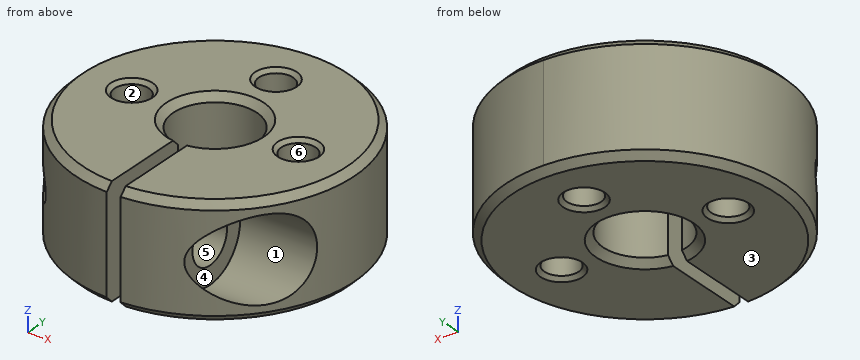
Autodesk Inventor part; units mm, degrees
ref_plane "to_bolt_XY" through (4, -6, 0) normal (1, 0, 0) x (0, 0, -1)
ref_plane "to_bolt_YZ" through (4, -6, 0) normal (0, 0, -1) x (0, 1, 0)
ref_plane "to_bolt_ZX" through (4, -6, 0) normal (0, 1, 0) x (1, 0, 0)
sketch "Sketch_14" plane through (0, 0, 0) normal (1, 0, 0) x (0, 1, 0)
  line L0 (0, -4) -> (0, 4)
  line L1 (0, 4) -> (9.5, 4)
  line L2 (9.5, 4) -> (10, 3.5)
  line L3 (10, 3.5) -> (10, -3.5)
  line L4 (10, -3.5) -> (9.5, -4)
  line L5 (9.5, -4) -> (0, -4)
  line L6 (0, -4) -> (0, 4)
revolve "Revolution1" add sketch "Sketch_14" angle 360 about axis through (0, 0, -4) along (0, 0, -1)
sketch "Sketch_15" plane through (0, 0, 0) normal (1, 0, 0) x (0, 1, 0)
  line L0 (0, -4) -> (0, 4)
  line L1 (0, 4) -> (3.5, 4)
  line L2 (3.5, 4) -> (3, 3.5)
  line L3 (3, 3.5) -> (3, -3.5)
  line L4 (3, -3.5) -> (3.5, -4)
  line L5 (3.5, -4) -> (0, -4)
  line L6 (0, -4) -> (0, 4)
revolve "Revolution2" cut sketch "Sketch_15" angle 360 about axis through (0, 0, -4) along (0, 0, -1)
sketch "Sketch_16" plane through (0, 0, 0) normal (0, 0, 1) x (1, 0, 0)
  arc A0 (-0.5, -10.9886) -> (0.5, -10.9886) centre (0, 0) ccw
  line L0 (0.5, -10.9886) -> (0.5, 0)
  line L1 (0.5, 0) -> (-0.5, 0)
  line L2 (-0.5, 0) -> (-0.5, -10.9886)
extrude "Extrusion1" cut sketch "Sketch_16" along normal mid plane 8
sketch "Sketch_18" plane through (6, 0, 0) normal (1, 0, 0) x (0, 0, -1)
  line L0 (4, 0) -> (-4, 0)
  line L1 (-4, 0) -> (-4, 1.5)
  line L2 (-4, 1.5) -> (-3.7295, 1.2295)
  line L3 (-3.7295, 1.2295) -> (3.7295, 1.2295)
  line L4 (3.7295, 1.2295) -> (4, 1.5)
  line L5 (4, 1.5) -> (4, 0)
  line L6 (4, 0) -> (-4, 0)
revolve "Revolution3" cut sketch "Sketch_18" angle 360 about axis through (6, 0, -4) along (0, 0, -1)
thread "Thread1"
sketch "Sketch_20" plane through (-6, 0, 0) normal (1, 0, 0) x (0, 0, -1)
  line L0 (4, 0) -> (-4, 0)
  line L1 (-4, 0) -> (-4, 1.5)
  line L2 (-4, 1.5) -> (-3.7295, 1.2295)
  line L3 (-3.7295, 1.2295) -> (3.7295, 1.2295)
  line L4 (3.7295, 1.2295) -> (4, 1.5)
  line L5 (4, 1.5) -> (4, 0)
  line L6 (4, 0) -> (-4, 0)
revolve "Revolution4" cut sketch "Sketch_20" angle 360 about axis through (-6, 0, -4) along (0, 0, -1)
thread "Thread2"
sketch "Sketch_22" plane through (0, 6, 0) normal (0, 1, 0) x (1, 0, 0)
  line L0 (0, 4) -> (0, -4)
  line L1 (0, -4) -> (-1.5, -4)
  line L2 (-1.5, -4) -> (-1.2295, -3.7295)
  line L3 (-1.2295, -3.7295) -> (-1.2295, 3.7295)
  line L4 (-1.2295, 3.7295) -> (-1.5, 4)
  line L5 (-1.5, 4) -> (0, 4)
  line L6 (0, 4) -> (0, -4)
revolve "Revolution5" cut sketch "Sketch_22" angle 360 about axis through (0, 6, -4) along (0, 0, -1)
thread "Thread3"
sketch "Sketch_23" plane through (0, -6, 0) normal (0, 1, 0) x (1, 0, 0)
  line L0 (10, 0) -> (0, 0)
  line L1 (0, 0) -> (0, 1.7)
  line L2 (0, 1.7) -> (4, 1.7)
  line L3 (4, 1.7) -> (4, 3)
  line L4 (4, 3) -> (10, 3)
  line L5 (10, 3) -> (10, 0)
  line L6 (10, 0) -> (0, 0)
revolve "Revolution6" cut sketch "Sketch_23" angle 360 about axis through (10, -6, 0) along (1, 0, 0)
sketch "Sketch_25" plane through (0, 0, 0) normal (0, 0, 1) x (1, 0, 0)
  line L0 (-0.5, -6) -> (-8.9303, -6)
  line L1 (-8.9303, -6) -> (-8.9303, -4.7705)
  line L2 (-8.9303, -4.7705) -> (-0.7705, -4.7705)
  line L3 (-0.7705, -4.7705) -> (-0.5, -4.5)
  line L4 (-0.5, -4.5) -> (-0.5, -6)
  line L5 (-0.5, -6) -> (-8.9303, -6)
revolve "Revolution7" cut sketch "Sketch_25" angle 360 about axis through (-0.5, -6, 0) along (1, 0, 0)
thread "Thread4"
ref_plane "to_bolt_XY" through (4, -6, 0) normal (1, 0, 0) x (0, 0, -1)
ref_plane "to_bolt_YZ" through (4, -6, 0) normal (0, 0, -1) x (0, 1, 0)
ref_plane "to_bolt_ZX" through (4, -6, 0) normal (0, 1, 0) x (1, 0, 0)
properties part number "SCSTR6-8b" material "鋼、炭素鋼"
Verification items for the finished model (mm, model axes). Face numbers are marked on the shaded views. A direction names the side the tool comes from. Coordinates: 2 decimals unless noted, no trailing zeros.
Item 1: Section check A-A, the plane x = -1.75. Give the number of separate pieces and of enclosed holes in the cut face, then the cut area to 3 significant figures.
Filled in:
separate pieces: 2
enclosed holes: 1
area: 113 mm2
Item 2: Material ranges on L1, parallel to X at y = 0, z = 0; L2, parallel to Z at x = 5.5, y = -6; L3, parallel to Y at x = -0.75, z = -0.75, recorded low to high.
Filled in:
L1: x = -10 to -7.23, -4.77 to -3, 3 to 4.77, 7.23 to 10
L2: z = -4 to -3, 3 to 4
L3: y = -9.97 to -7, -5 to -2.9, 2.9 to 5.03, 6.97 to 9.97
Item 3: Access from +Z, -Z, +X, -X, +Y, -Y to the whole of each face (thin tool, end or side, straight path). Record for the marked faces 1 and 2.
Filled in:
face 1: +X
face 2: +Z, -Z
Item 4: Release check for a two-part mould opening along Z. For the marked faces 3, 4, 5 and 6 record: +Z half, -Z half, draft (parallel to the pull), parting line (faces both ways), or undercut.
Filled in:
face 3: -Z half
face 4: undercut
face 5: undercut
face 6: draft
Item 5: Depth check by flat-ended pin: pin 1 (2 mm diameter, centred on x = 5, z = 1.5, fed in from +Y); pin 2 (3 mm diameter, centred on y = -6, z = 0, fed in from -X); pin 3 (10 mm diameter, centred on x = -1, y = 2.5, fed in from +Z); pin 4 (2 mm diameter, centred on y = -8, z = -0.5, fed in from -X). Enter the tip coordinate at first touch or a pass-through.
Filled in:
pin 1: stops at y = 9.17
pin 2: stops at x = -8.93
pin 3: stops at z = 4
pin 4: stops at x = -7.12
